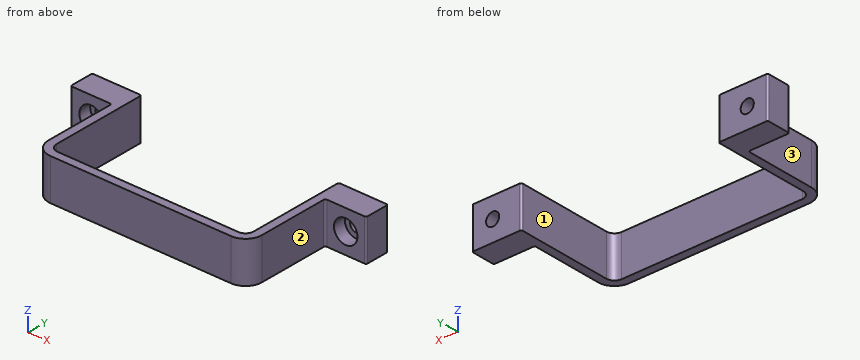
from build123d import *

# Parameters (mm, degrees)
PAD_DEPTH            = 10
SKETCH002_R          = 1.6
POCKET_DEPTH         = 6
SKETCH003_R          = 2.85
POCKET001_DEPTH      = 3
FILLET_R             = 0.4
BODY_PLACEMENT_ANGLE = 90


with BuildPart() as part:
    # Sketch → Pad (new body)
    with BuildSketch(Plane.XZ):
        with BuildLine():
            Line((-36, 0), (-36, -6))
            Line((-36, -6), (-26, -6))
            Line((-26, -6), (-26, -23.5))
            ThreePointArc((-26, -23.5), (-24.828427, -26.328427), (-22, -27.5))
            Line((-22, -27.5), (22, -27.5))
            ThreePointArc((22, -27.5), (24.828427, -26.328427), (26, -23.5))
            Line((26, -23.5), (26, -6))
            Line((26, -6), (36, -6))
            Line((36, -6), (36, 0))
            Line((36, 0), (24, 0))
            Line((24, 0), (24, -23.5))
            ThreePointArc((22, -25.5), (23.414214, -24.914214), (24, -23.5))
            Line((22, -25.5), (-22, -25.5))
            ThreePointArc((-24, -23.5), (-23.414214, -24.914214), (-22, -25.5))
            Line((-24, -23.5), (-24, 0))
            Line((-24, 0), (-36, 0))
        make_face()
    extrude(amount=-PAD_DEPTH)

    # Sketch002 (on Face4 of Pad) → Pocket (cut)
    with BuildSketch(Plane(origin=(0, 0, -6), x_dir=(1, 0, 0), z_dir=(0, 0, -1))):
        with Locations((-31, -5)):
            Circle(SKETCH002_R)
        with Locations((31, -5)):
            Circle(SKETCH002_R)
    extrude(amount=-POCKET_DEPTH, mode=Mode.SUBTRACT)

    # Sketch003 (on Face9 of Pocket) → Pocket001 (cut)
    with BuildSketch(Plane(origin=(0, 0, -6), x_dir=(1, 0, 0), z_dir=(0, 0, -1))):
        with Locations((-31, -5)):
            Circle(SKETCH003_R)
        with Locations((31, -5)):
            Circle(SKETCH003_R)
    extrude(amount=-POCKET001_DEPTH, mode=Mode.SUBTRACT)

    # Fillet
    fillet_edges = [part.edges().sort_by_distance(p)[0] for p in [
        (26, 5, -6),
        (36, 5, -6),
        (36, 5, 0),
        (24, 5, 0),
        (-24, 5, 0),
        (-36, 5, 0),
        (-36, 5, -6),
        (-26, 5, -6),
    ]]
    fillet(fillet_edges, radius=FILLET_R)


with BuildPart() as part_1:
    # Body placement: moved
    add(part.part.rotate(Axis((0, 0, 0), (-1, 0, 0)), BODY_PLACEMENT_ANGLE))


solid = part_1.part
Work out the finished part from the listing and answer in its coordinate system (mm). Face numbers are marked on the shaded views. A direction names the side the tool comes from. Give positions to 0.01 mm unless a question says otherwise; leave off trailing zeros. Loops run counter-clockwise (first coordinate to the right, second up) from the corner with the lowest first, then second, coordinate; pieces in that order, holes last. Notation, with made-up numbers: (-5, 44.5) - (10, 44.5) arc R14 ccw to (10, 50.5) - close; hole circle Ø10 at (85.25, -33.75). An arc over 180 degrees is marked (long way). Answer in a Markdown table with one row per item. Add a question column.
Q1. Each of these flat-tipped pins is pushed along its axis until it touches: P1, Ø5, axis at x = 9, z = -6, coming from the +Y side; P2, Ø1, axis at y = -12.5, z = -2, coming from the +X side; P3, Ø4.5, axis at x = 31, z = -5, coming from the -Y side. Where does it stop, or does it pass through?
Q2. Consider line 1 along X through (y, z) = (-23.25, -0.75); line 2 along Z through (x, y) = (-31, -4.85); line 3 along Z through (x, y) = (-31, -1.15). Determine where each line is inside the solid, lowest interval first.
Q3. The part is cut by section A-A (y = -21.25). Determine the outline of the cut face in (x, z), and give its area (3 significant figures).
Q4. The part is cut by section D-D (x = 18). Determine the outline of the cut face in (y, z).
Q5. The part is cut by section C-C (z = -5). State how many separate pieces and enclosed holes the cut face has, and give its area (3 significant figures).
Q6. A tool of negligible diameter and unlimited length cuts with its end or side. For the marked faces 1, 2 and 3, from which of +Z, -Z, +X, -X, +Y, -Y can it reach the whole face along a straight path? Write none if from no direction.
Q7. The part is cut by section B-B (x = -31). Determine the outline of the cut face in (y, z).
Solution:
| question | item | result |
|---|---|---|
| 1 | P1 | stops at y = -25.5 |
| 1 | P2 | stops at x = 26 |
| 1 | P3 | stops at y = -3 |
| 2 | line 1 | x = -26 to -24, 24 to 26 |
| 2 | line 2 | z = -10 to -7.85, -2.15 to 0 |
| 2 | line 3 | z = -10 to -6.6, -3.4 to 0 |
| 3 | outline | (-26, -10) - (-24, -10) - (-24, 0) - (-26, 0) - close; (24, -10) - (26, -10) - (26, 0) - (24, 0) - close |
| 3 | area | 40.0 mm² |
| 4 | outline | (-27.5, -10) - (-25.5, -10) - (-25.5, 0) - (-27.5, 0) - close |
| 5 | separate pieces | 3 |
| 5 | enclosed holes | 0 |
| 5 | area | 267 mm² |
| 6 | face 1 | +Z, -Z, +Y |
| 6 | face 2 | +Z, -Z, +X, -Y |
| 6 | face 3 | +Z, -Z, -X, -Y |
| 7 | outline | (-6, -10) - (0, -10) - (0, -6.6) - (-3, -6.6) - (-3, -7.85) - (-6, -7.85) - close; (-6, -2.15) - (-3, -2.15) - (-3, -3.4) - (0, -3.4) - (0, 0) - (-6, 0) - close |
